```python
from build123d import *

# Parameters (mm, degrees)
SKETCH_1_R          = 3
SKETCH_1_R_2        = 1.5
EXTRUDE_1_DEPTH     = 5
EXTRUDE_2_DEPTH     = 5
SKETCH_4_R          = 1.5
CUT_EXTRUDE_1_DEPTH = 144.265487819
EXTRUDE_START       = -5
EXTRUDE_3_DEPTH     = 5
CUT_EXTRUDE_2_DEPTH = 144.265487819
SKETCH_7_R          = 1.6
CUT_EXTRUDE_3_DEPTH = 144.265487819
FILLET_1_R          = 2


with BuildPart() as part:
    # 草图1 → 凸台-拉伸1 (new body)
    with BuildSketch(Plane.XY):
        with BuildLine():
            Line((-3.933140204, 6.966376973), (90, 60))
            Line((90, 60), (130, 60))
            Line((130, 60), (130, 30))
            Line((130, 30), (92, 30))
            Line((92, 30), (3.100465808, -7.374761811))
            ThreePointArc((3.100465808, -7.374761811), (-7.182645896, -3.522725923), (-3.933140204, 6.966376973))
        make_face()
        Circle(SKETCH_1_R, mode=Mode.SUBTRACT)
        with Locations((95, 55)):
            Circle(SKETCH_1_R_2, mode=Mode.SUBTRACT)
        with Locations((125, 55)):
            Circle(SKETCH_1_R_2, mode=Mode.SUBTRACT)
        with Locations((125, 35)):
            Circle(SKETCH_1_R_2, mode=Mode.SUBTRACT)
        with Locations((95, 35)):
            Circle(SKETCH_1_R_2, mode=Mode.SUBTRACT)
    extrude(amount=EXTRUDE_1_DEPTH)

    # 草图3 → 凸台-拉伸2 (add)
    with BuildSketch(Plane.XY.offset(5)):
        Polygon((81.144001216, 55), (20, 55), (20, 20.478766027), align=None)
    extrude(amount=-EXTRUDE_2_DEPTH)

    # 草图4 → 切除-拉伸1 (cut, through all)
    with BuildSketch(Plane.XY.offset(5)):
        with Locations((25, 52)):
            Circle(SKETCH_4_R)
        with Locations((45, 52)):
            Circle(SKETCH_4_R)
    extrude(amount=-CUT_EXTRUDE_1_DEPTH, mode=Mode.SUBTRACT)

    # 草图6 → 凸台-拉伸3 (add)
    with BuildSketch(Plane.XY.offset(5).offset(EXTRUDE_START)):
        with BuildLine():
            Line((-7.074049095, 3.736017853), (20, 55))
            Line((20, 55), (20, 20.478766027))
            Line((20, 20.478766027), (-3.933140204, 6.966376973))
            ThreePointArc((-3.933140204, 6.966376973), (-5.735709118, 5.576884517), (-7.074049095, 3.736017853))
        make_face()
    extrude(amount=EXTRUDE_3_DEPTH)

    # 草图5 → 切除-拉伸2 (cut, through all)
    with BuildSketch(Plane.XY.offset(5)):
        with BuildLine():
            Line((105, 52), (115, 52))
            ThreePointArc((115, 52), (122, 45), (115, 38))
            Line((115, 38), (105, 38))
            ThreePointArc((105, 38), (98, 45), (105, 52))
        make_face()
        with BuildLine():
            Line((25.605401824, 44.200503347), (15.042800964, 24.200503347))
            ThreePointArc((15.042800964, 24.200503347), (15.293877797, 22.454192152), (17.032531201, 22.154647985))
            Line((17.032531201, 22.154647985), (57.595132061, 42.154647985))
            ThreePointArc((57.595132061, 42.154647985), (58.392612512, 43.840567158), (56.93178603, 45))
            Line((56.93178603, 45), (26.93178603, 45))
            ThreePointArc((26.93178603, 45), (26.157433081, 44.784670195), (25.605401824, 44.200503347))
        make_face()
    extrude(amount=-CUT_EXTRUDE_2_DEPTH, mode=Mode.SUBTRACT)

    # 草图7 → 切除-拉伸3 (cut, through all)
    with BuildSketch(Plane.XY.offset(5)):
        with Locations((10, 18)):
            Circle(SKETCH_7_R)
        with Locations((30, 18)):
            Circle(SKETCH_7_R)
    extrude(amount=-CUT_EXTRUDE_3_DEPTH, mode=Mode.SUBTRACT)

    # 圆角1
    fillet_1_edges = [part.edges().sort_by_distance(p)[0] for p in [
        (20, 55, 2.5),
    ]]
    fillet(fillet_1_edges, radius=FILLET_1_R)


solid = part.part
```
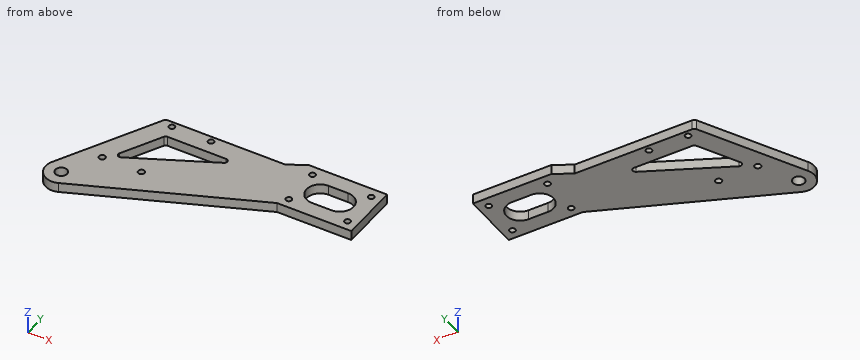
Geometry: final body of the model. Coordinates: model frame, mm. Coordinates: 2 decimals unless noted, no trailing zeros. Write each loop counter-clockwise with the first axis right and the second up, starting at its lowest first coordinate (ties: lowest second). Pieces come first, ordered by that corner, then holes. Notation, with made-up numbers: M 25,21 L 74,21 A28 cw 74,58 Z; hole C -31,55 d3. An arc over 180 degrees is marked long. Use CSV: the item, a comma, the result in double quotes. Start each with the question number.
1. Ray query, probe 1 along X at (y, z) = (36, 1.75); probe 2 along Y at (x, z) = (112, 1.05); probe 3 along Y at (x, z) = (-0.5, 0.75). Return the intervals inside material, ascending.
2. Cut plane A-A on x = 112. Return the cut outline in (y, z), plus the area to 3 significant figures.
3. Cut plane B-B on z = 1.85. Count the separate pieces of the cut face and the enclosed holes in it, plus the area to 3 significant figures.
4. First-contact query: P1, Ø2.5, axis at x = 43, z = 2.5, coming from the -Y side; P2, Ø3.5, axis at x = 0, y = 0, coming from the +Z side; P3, Ø3.5, axis at x = 125, y = 35, coming from the -Z side; P4, Ø1, axis at x = 26, z = 2, coming from the +Y side. Flat tips, straight axial feed; report the tip coordinate or a pass-through.
5. Cut plane C-C on y = 26. Return the cut outline in (x, z).
6. Cut plane D-D on x = 45. Return the cut outline in (y, z).
Entries:
1,probe 1,"9.97 to 21.27, 45.11 to 93.88, 96.12 to 123.88, 126.12 to 130"
1,probe 2,"30 to 38, 52 to 60"
1,probe 3,"-7.98 to -2.96, 2.96 to 16.18"
2,outline,"M 30,0 L 38,0 L 38,5 L 30,5 Z; M 52,0 L 60,0 L 60,5 L 52,5 Z"
2,area,"80.0 mm²"
3,separate pieces,"1"
3,enclosed holes,"11"
3,area,"4,160 mm²"
4,P1,"y = 8.87"
4,P2,"through"
4,P3,"z = 0"
4,P4,"y = 55"
5,outline,"M 4.68,0 L 15.99,0 L 15.99,5 L 4.68,5 Z; M 24.83,0 L 82.49,0 L 82.49,5 L 24.83,5 Z"
6,outline,"M 10.24,0 L 35.94,0 L 35.94,5 L 10.24,5 Z; M 45,0 L 50.5,0 L 50.5,5 L 45,5 Z; M 53.5,0 L 55,0 L 55,5 L 53.5,5 Z"
